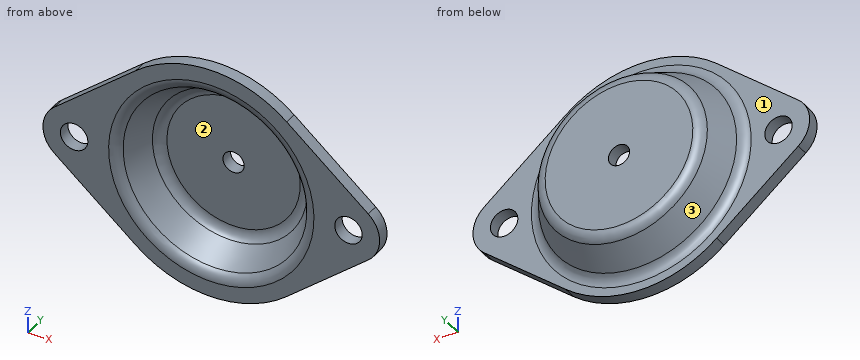
```python
from build123d import *

# Parameters (mm, degrees)
ZAOKR_GLENIE1_R                 = 5
SZKIC2_R                        = 5.5
WYTNIJ_WYCI_GNI_CIE1_DEPTH      = 98.532046016
OTW_R_GWINTOWANY_M101_D         = 8.5
OTW_R_GWINTOWANY_M101_DEPTH     = 17.5
OTW_R_GWINTOWANY_M101_TIP       = 2.553657631
WYTNIJ_WYCI_GNI_CIE2_DEPTH      = 97.63074045
WYTNIJ_WYCI_GNI_CIE2_DEPTH_BACK = 97.63074045
SZKIC5_OUTSIDE_W                = 175.392
SZKIC5_OUTSIDE_H                = 175.392


with BuildPart() as part:
    # Szkic1 → Obrót1 (revolve)
    with BuildSketch(Plane.XY, mode=Mode.PRIVATE) as obr_t1_sk:
        Polygon((0, 0), (-32.5, 0), (-41.160254038, -15), (-67.5, -15), (-67.5, -20), (-38.273502692, -20), (-29.613248654, -5), (0, -5), align=None)
    revolve(obr_t1_sk.sketch.rotate(Axis((0, 100.333333333, 0), (0, -1, 0)), 270), axis=Axis((0, 100.333333333, 0), (0, -1, 0)))

    # Zaokrąglenie1
    zaokr_glenie1_edges = [part.edges().sort_by_distance(p)[0] for p in [
        (0, -5, -29.613248654),
        (0, -20, -38.273502692),
        (0, -15, -41.160254038),
        (0, 0, -32.5),
    ]]
    fillet(zaokr_glenie1_edges, radius=ZAOKR_GLENIE1_R)

    # Szkic2 → Wytnij-wyciągnięcie1 (cut, through all)
    with BuildSketch(Plane(origin=(0, 0, 0), x_dir=(1, 0, 0), z_dir=(0, 1, 0))):
        with Locations(Location((-55, 0, 0), (0, 0, 270))):
            Circle(SZKIC2_R)
        with Locations(Location((55, 0, 0), (0, 0, 270))):
            Circle(SZKIC2_R)
    extrude(amount=-WYTNIJ_WYCI_GNI_CIE1_DEPTH, mode=Mode.SUBTRACT)

    # Otwór gwintowany M101
    with Locations(Plane(origin=(0, 0, 0), x_dir=(1, 0, 0), z_dir=(0, 1, 0))):
        with Locations((0, 0)):
            Hole(OTW_R_GWINTOWANY_M101_D / 2, depth=OTW_R_GWINTOWANY_M101_DEPTH)
            with Locations((0, 0, -(OTW_R_GWINTOWANY_M101_DEPTH + OTW_R_GWINTOWANY_M101_TIP / 2))):  # 118° drill point
                Cone(0, OTW_R_GWINTOWANY_M101_D / 2, OTW_R_GWINTOWANY_M101_TIP, mode=Mode.SUBTRACT)

    # Szkic5 outside → Wytnij-wyciągnięcie2 (cut, two sides: drawn at the far end of the back side and taken through both)
    with BuildSketch(Plane(origin=(0, -15, 0), x_dir=(1, 0, 0), z_dir=(0, 1, 0)).offset(-WYTNIJ_WYCI_GNI_CIE2_DEPTH_BACK)):
        Rectangle(SZKIC5_OUTSIDE_W, SZKIC5_OUTSIDE_H)
        with BuildLine():
            Line((62.954545455, 9.642365198), (30.227272727, 36.640987752))
            ThreePointArc((30.227272727, 36.640987752), (0, 47.5), (-30.227272727, 36.640987752))
            Line((-30.227272727, 36.640987752), (-62.954545455, 9.642365198))
            ThreePointArc((-62.954545455, 9.642365198), (-67.5, 0), (-62.954545455, -9.642365198))
            Line((-62.954545455, -9.642365198), (-30.227272727, -36.640987752))
            ThreePointArc((-30.227272727, -36.640987752), (0, -47.5), (30.227272727, -36.640987752))
            Line((30.227272727, -36.640987752), (62.954545455, -9.642365198))
            ThreePointArc((62.954545455, -9.642365198), (67.5, 0), (62.954545455, 9.642365198))
        make_face(mode=Mode.SUBTRACT)
    extrude(amount=WYTNIJ_WYCI_GNI_CIE2_DEPTH + WYTNIJ_WYCI_GNI_CIE2_DEPTH_BACK, mode=Mode.SUBTRACT)


solid = part.part
```
Work out the finished part from the listing and answer in its coordinate system (mm). Face numbers are marked on the shaded views. Coordinates: 2 decimals unless noted, no trailing zeros. Write each loop counter-clockwise with the first axis right and the second up, starting at its lowest first coordinate (ties: lowest second). Pieces come first, ordered by that corner, then holes.
Q1. A cutting plane is placed at A-A, the plane x = 0. Give the vertices of the cut face in (y, z).
Q2. Each of these flat-tipped pins is pushed along its axis until it touches: pin 1 Ø8 at (x, z) = (-4, -18) entering from +Y; pin 2 Ø5 at (x, y) = (-27, -7) entering from -Z; pin 3 Ø8 at (x, y) = (-47, -17) entering from -Z; pin 4 Ø14.5 at (x, z) = (55, 0) entering from +Y. Where does it stop, or does it pass through?
Q3. A cutting plane is placed at B-B, the plane z = 0. State how many separate pieces and enclosed holes the cut face has, then the cut area to 3 significant figures.
Q4. Find the intervals of material crossed by line 1 (X direction, y = -18.9, z = 0); line 2 (X direction, y = -16.1, z = 0); line 3 (Y direction, x = 37, z = 28), in increasing order.
Q5. Determine the mould class of the marked faces 1, 2 and 3 for opening direction X: released by +X, released by -X, zero draft, split by the parting line, or undercut.
Q6. A cutting plane is placed at C-C, the plane x = -55. Give the vertices of the cut face in (y, z).
Findings below:
1. outline: (-20, -47.5) - (-15, -47.5) - (-15, -44.05) arc R5 cw to (-12.5, -39.72) - (-2.5, -33.94) arc R5 ccw to (0, -29.61) - (0, -4.25) - (-5, -4.25) - (-5, -26.73) arc R5 cw to (-7.5, -31.06) - (-17.5, -36.83) arc R5 ccw to (-20, -41.16) - close; (-20, 41.16) arc R5 ccw to (-17.5, 36.83) - (-7.5, 31.06) arc R5 cw to (-5, 26.73) - (-5, 4.25) - (0, 4.25) - (0, 29.61) arc R5 ccw to (-2.5, 33.94) - (-12.5, 39.72) arc R5 cw to (-15, 44.05) - (-15, 47.5) - (-20, 47.5) - close
2. pin 1: stops at y = 0
2. pin 2: stops at z = -27.83
2. pin 3: stops at z = -26.1
2. pin 4: stops at y = -15
3. separate pieces: 4
3. enclosed holes: 0
3. area: 609 mm2
4. line 1: x = -67.5 to -60.5, -49.5 to -38.03, 38.03 to 49.5, 60.5 to 67.5
4. line 2: x = -67.5 to -60.5, -49.5 to -36.02, 36.02 to 49.5, 60.5 to 67.5
4. line 3: y = -20 to -15
5. face 1: zero draft
5. face 2: undercut
5. face 3: split by the parting line
6. outline: (-20, -16.2) - (-15, -16.2) - (-15, -5.5) - (-20, -5.5) - close; (-20, 5.5) - (-15, 5.5) - (-15, 16.2) - (-20, 16.2) - close
